Read the model definition and answer for the solid it produces. Units are mm, in the model's axes. A direction names the side the tool comes from. Give positions to 0.01 mm unless a question says otherwise; leave off trailing zeros. Loops run counter-clockwise (first coordinate to the right, second up) from the corner with the lowest first, then second, coordinate; pieces in that order, holes last.
(1) Find section D-D, the plane y = -12. Write down the section's boundary in (x, z).
(2) Find section C-C, the plane x = -10.5. Write down the section's boundary in (y, z), then the cut area to 3 significant figures.
(3) Determine the mould class of faces 1 (the face through (-11.684, -42, 1)), 2 (the face through (0, -43.111, 1)), 3 (the face through (-7.11, -29.86, 0.83)) for opening direction Y: pulls with the +Y half, pulls with the -Y half, needs draft (parallel to the pull), parting line crosses it, or undercut.
(4) Each of these flat-tipped pins is pushed along its axis until it touches: P1, Ø1, axis at y = -19, z = 1, coming from the -X side; P2, Ø0.5, axis at y = 3, z = 0.5, coming from the -X side; P3, Ø2, axis at x = -5, y = -7, coming from the +Z side. Where does it stop, or does it pass through?
(5) Which of the six approach directions +Z, -Z, +X, -X, +Y, -Y give full straight-line access (tool end or side, diameter ignored) to faces 4 (the face through (7.1, 28.1, 0.8)), 5 (the face through (-7.23, 28.41, 0.83)), 6 (the face through (0, 41.318, 1))?
(6) Straight lines are drawn through the part: probe 1 along X at (y, z) = (11, 0.55); probe 2 along Y at (x, z) = (-8, 0.7); probe 3 along Y at (x, z) = (9.75, 0.9). For each, find the intervals that lie inside material, in ascending order.
(7) Find section B-B, the plane z = 0.5. Write down the section's boundary in (x, y).
(8) Find section A-A, the plane x = 5.5. Write down the section's boundary in (y, z), then the cut area to 3 significant figures.
```python
from build123d import *

# Parameters (mm, degrees)
F0_W     = 2.6543
F0_H     = 36.782036
F1_DEPTH = 1.6764


with BuildPart() as f1:
    # F0 (on Top) → F1 (new body)
    with BuildSketch(Plane.XY):
        Polygon((0, 41.318396), (0, 17.543996), (2.6543, 17.543996), (11.684, 38.981596), (11.684, 41.318396), align=None)
        Polygon((-2.6543, 17.543996), (0, 17.543996), (0, 41.318396), (-11.684, 41.318396), (-11.684, 38.981596), align=None)
        with Locations((1.32715, -0.847022)):
            Rectangle(F0_W, F0_H)
        with Locations((-1.32715, -0.847022)):
            Rectangle(F0_W, F0_H)
        Polygon((0, -19.336804), (0, -19.23804), (-2.6543, -19.23804), (-11.684, -40.774404), (-11.684, -43.111204), (0, -43.111204), align=None)
        Polygon((2.6543, -19.23804), (0, -19.23804), (0, -19.336804), (0, -43.111204), (11.684, -43.111204), (11.684, -40.774404), align=None)
    extrude(amount=F1_DEPTH)


solid = f1.part
```
Entries:
1. outline: (-2.65, 0) - (2.65, 0) - (2.65, 1.68) - (-2.65, 1.68) - close
2. outline: (-43.11, 0) - (-37.95, 0) - (-37.95, 1.68) - (-43.11, 1.68) - close; (36.17, 0) - (41.32, 0) - (41.32, 1.68) - (36.17, 1.68) - close
2. area: 17.3 mm2
3. face 1: needs draft
3. face 2: pulls with the -Y half
3. face 3: undercut
4. P1: stops at x = -2.76
4. P2: stops at x = -2.65
4. P3: passes through
5. face 4: +Z, -Z, +X
5. face 5: +Z, -Z, -X
5. face 6: +Z, -Z, +X, -X, +Y
6. probe 1: x = -2.65 to 2.65
6. probe 2: y = -43.11 to -31.99, 30.24 to 41.32
6. probe 3: y = -43.11 to -36.16, 34.39 to 41.32
7. outline: (-11.68, -43.11) - (11.68, -43.11) - (11.68, -40.77) - (2.65, -19.24) - (2.65, 17.54) - (11.68, 38.98) - (11.68, 41.32) - (-11.68, 41.32) - (-11.68, 38.98) - (-2.65, 17.54) - (-2.65, -19.24) - (-11.68, -40.77) - close
8. outline: (-43.11, 0) - (-26.03, 0) - (-26.03, 1.68) - (-43.11, 1.68) - close; (24.3, 0) - (41.32, 0) - (41.32, 1.68) - (24.3, 1.68) - close
8. area: 57.2 mm2
